For this review, take the finished solid that the model builds, in its own axes (mm). A direction names the side the tool comes from. Coordinates: 2 decimals unless noted, no trailing zeros. Loops run counter-clockwise (first coordinate to the right, second up) from the corner with the lowest first, then second, coordinate; pieces in that order, holes last. Notation, with made-up numbers: (77, -35) -> (95, -35) arc R28 cw to (95, -14) -> close; hole circle Ø8 at (-34.5, 38). An arc over 180 degrees is marked (long way). Use a Markdown table: item, result.
from build123d import *

# Parameters (mm, degrees)
SKETCH001_W     = 298
SKETCH001_H     = 108
SKETCH001_W_2   = 287
SKETCH001_H_2   = 97
PAD_DEPTH       = 9.5
SKETCH002_W     = 295
SKETCH002_H     = 105
POCKET_DEPTH    = 1.7
SKETCH003_W     = 80
SKETCH003_H     = 4
POCKET001_DEPTH = 2.8
SKETCH004_W     = 4
SKETCH004_H     = 32.5
POCKET002_DEPTH = 2.8
FILLET_R        = 1.5
FILLET001_R     = 1
FILLET002_R     = 1
FILLET003_R     = 1
FILLET004_R     = 1


with BuildPart() as part:
    # Sketch001 → Pad (new body)
    with BuildSketch(Plane.XY):
        Rectangle(SKETCH001_W, SKETCH001_H)
        Rectangle(SKETCH001_W_2, SKETCH001_H_2, mode=Mode.SUBTRACT)
    extrude(amount=PAD_DEPTH)

    # Sketch002 (on Face9 of Pad) → Pocket (cut)
    with BuildSketch(Plane(origin=(0, 0, 0), x_dir=(1, 0, 0), z_dir=(0, 0, -1))):
        Rectangle(SKETCH002_W, SKETCH002_H)
    extrude(amount=-POCKET_DEPTH, mode=Mode.SUBTRACT)

    # Sketch003 (on Face15 of Pocket) → Pocket001 (cut)
    with BuildSketch(Plane(origin=(0, 0, 1.7), x_dir=(1, 0, 0), z_dir=(0, 0, -1))):
        with Locations((-95, 50.5)):
            Rectangle(SKETCH003_W, SKETCH003_H)
        with Locations((0, 50.5)):
            Rectangle(SKETCH003_W, SKETCH003_H)
        with Locations((95, 50.5)):
            Rectangle(SKETCH003_W, SKETCH003_H)
        with Locations((-95, -50.5)):
            Rectangle(SKETCH003_W, SKETCH003_H)
        with Locations((0, -50.5)):
            Rectangle(SKETCH003_W, SKETCH003_H)
        with Locations((95, -50.5)):
            Rectangle(SKETCH003_W, SKETCH003_H)
    extrude(amount=-POCKET001_DEPTH, mode=Mode.SUBTRACT)

    # Sketch004 (on Face15 of Pocket001) → Pocket002 (cut)
    with BuildSketch(Plane(origin=(0, 0, 1.7), x_dir=(1, 0, 0), z_dir=(0, 0, -1))):
        with Locations((145.5, 23.75)):
            Rectangle(SKETCH004_W, SKETCH004_H)
        with Locations((145.5, -23.75)):
            Rectangle(SKETCH004_W, SKETCH004_H)
        with Locations((-145.5, 23.75)):
            Rectangle(SKETCH004_W, SKETCH004_H)
        with Locations((-145.5, -23.75)):
            Rectangle(SKETCH004_W, SKETCH004_H)
    extrude(amount=-POCKET002_DEPTH, mode=Mode.SUBTRACT)

    # Fillet
    fillet_edges = [part.edges().sort_by_distance(p)[0] for p in [
        (149, -54, 4.75),
        (-149, -54, 4.75),
        (-149, 54, 4.75),
        (149, 54, 4.75),
    ]]
    fillet(fillet_edges, radius=FILLET_R)

    # Fillet001
    fillet001_edges = [part.edges().sort_by_distance(p)[0] for p in [
        (0, 54, 9.5),
    ]]
    fillet(fillet001_edges, radius=FILLET001_R)

    # Fillet002
    fillet002_edges = [part.edges().sort_by_distance(p)[0] for p in [
        (-147.5, 52.5, 0.85),
        (-147.5, -52.5, 0.85),
        (147.5, -52.5, 0.85),
        (147.5, 52.5, 0.85),
    ]]
    fillet(fillet002_edges, radius=FILLET002_R)

    # Fillet003
    fillet003_edges = [part.edges().sort_by_distance(p)[0] for p in [
        (143.5, 40, 3.1),
        (135, 48.5, 3.1),
        (55, 48.5, 3.1),
        (40, 48.5, 3.1),
        (-55, 48.5, 3.1),
        (-40, 48.5, 3.1),
        (-135, 48.5, 3.1),
        (-143.5, 40, 3.1),
        (-143.5, -7.5, 3.1),
        (143.5, -7.5, 3.1),
        (143.5, 7.5, 3.1),
        (143.5, -40, 3.1),
        (135, -48.5, 3.1),
        (40, -48.5, 3.1),
        (-55, -48.5, 3.1),
        (-143.5, 7.5, 3.1),
        (-143.5, -40, 3.1),
        (-135, -48.5, 3.1),
        (-40, -48.5, 3.1),
        (55, -48.5, 3.1),
    ]]
    fillet(fillet003_edges, radius=FILLET003_R)

    # Fillet004
    fillet004_edges = [part.edges().sort_by_distance(p)[0] for p in [
        (-143.5, -48.5, 5.6),
        (143.5, 48.5, 5.6),
        (143.5, -48.5, 5.6),
        (-143.5, 48.5, 5.6),
    ]]
    fillet(fillet004_edges, radius=FILLET004_R)


solid = part.part
(1) For faces 4 (the face through (143.5, -1, 6)), 5 (the face through (-149, -1, 4)), 6 (the face through (-144, -48, 1.7)), list the 3-axis set-ups (+Z, -Z, +X, -X, +Y, -Y) from which the entire face can be reached by the end or side of a thin tool; tool diameter is ignored.
Found:
| item | result |
|---|---|
| face 4 | +Z, -Z |
| face 5 | +Z, -Z, -X, +Y, -Y |
| face 6 | -Z |
(2) Take a section at A-A on y = 44. Write out the cut boundary in (x, z), plus the area to 3 significant figures.
Found:
| item | result |
|---|---|
| outline | (-149, 0) -> (-147.5, 0) -> (-147.5, 1.7) -> (-143.5, 1.7) -> (-143.5, 9.5) -> (-148, 9.5) arc R1 ccw to (-149, 8.5) -> close; (143.5, 1.7) -> (147.5, 1.7) -> (147.5, 0) -> (149, 0) -> (149, 8.5) arc R1 ccw to (148, 9.5) -> (143.5, 9.5) -> close |
| area | 90.5 mm^2 |
(3) Take a section at C-C on z = 6.5. Write out the cut boundary in (x, y).
Found:
| item | result |
|---|---|
| outline | (-149, -52.5) arc R1.5 ccw to (-147.5, -54) -> (147.5, -54) arc R1.5 ccw to (149, -52.5) -> (149, 52.5) arc R1.5 ccw to (147.5, 54) -> (-147.5, 54) arc R1.5 ccw to (-149, 52.5) -> close; hole (-143.5, -47.5) arc R1 ccw to (-142.5, -48.5) -> (142.5, -48.5) arc R1 ccw to (143.5, -47.5) -> (143.5, 47.5) arc R1 ccw to (142.5, 48.5) -> (-142.5, 48.5) arc R1 ccw to (-143.5, 47.5) -> close |
(4) Mouldability with a two-part tool opening along Y and no side actions: class faces 1 (the face through (-1, 51, 9.5)), 2 (the face through (143, -49, 1.7)), 3 (the face through (-2, -54, 4)) as pulls with the +Y half, pulls with the -Y half, needs draft (parallel to the pull), parting line crosses it, or undercut.
Found:
| item | result |
|---|---|
| face 1 | needs draft |
| face 2 | undercut |
| face 3 | pulls with the -Y half |
(5) For pin 1 Ø1.2 at (x, y) = (-45.5, -50) entering from -Z; pin 2 Ø2 at (x, y) = (17, 50.5) entering from -Z, all flat-tipped, find the tip position at first contact; note any pin that passes through.
Found:
| item | result |
|---|---|
| pin 1 | stops at z = 1.7 |
| pin 2 | stops at z = 4.5 |
(6) For line 1 along Y through (x, z) = (-20.5, 2); line 2 along Y through (x, z) = (133, 4.75); line 3 along X through (y, z) = (-34.5, 1.25), list the stretches that pass through material, from the lowest coordinate up.
Found:
| item | result |
|---|---|
| line 1 | y = -54 to -52.5, 52.5 to 54 |
| line 2 | y = -54 to -48.5, 48.5 to 54 |
| line 3 | x = -149 to -147.5, 147.5 to 149 |
(7) Take a section at B-B on x = -51. Write out the cut boundary in (y, z), plus the area to 3 significant figures.
Found:
| item | result |
|---|---|
| outline | (-54, 0) -> (-52.5, 0) -> (-52.5, 1.7) -> (-48.5, 1.7) -> (-48.5, 9.5) -> (-53, 9.5) arc R1 ccw to (-54, 8.5) -> close; (48.5, 1.7) -> (52.5, 1.7) -> (52.5, 0) -> (54, 0) -> (54, 8.5) arc R1 ccw to (53, 9.5) -> (48.5, 9.5) -> close |
| area | 90.5 mm^2 |
